from build123d import *

# Parameters (mm, degrees)
SKETCH1_W           = 18
SKETCH1_H           = 18
SKETCH1_R           = 5
BOSS_EXTRUDE1_DEPTH = 18
SKETCH2_R           = 5
CUT_EXTRUDE1_DEPTH  = 3


with BuildPart() as part:
    # Sketch1 → Boss-Extrude1 (new body)
    with BuildSketch(Plane.XY):
        Rectangle(SKETCH1_W, SKETCH1_H)
        Circle(SKETCH1_R, mode=Mode.SUBTRACT)
    extrude(amount=BOSS_EXTRUDE1_DEPTH)

    # Sketch2 → Cut-Extrude1 (cut)
    with BuildSketch(Plane(origin=(9, 0, 0), x_dir=(0, 0, -1), z_dir=(1, 0, 0))):
        with Locations(Location((-9, 0, 0), (0, 0, 90))):
            Circle(SKETCH2_R)
    cut_extrude1 = extrude(amount=-CUT_EXTRUDE1_DEPTH, mode=Mode.SUBTRACT)

    # Mirror1: Cut-Extrude1 across plane
    add(cut_extrude1.mirror(Plane(origin=(0, 0, 0), x_dir=(0, 0, 1), z_dir=(1, 0, 0))), mode=Mode.SUBTRACT)


solid = part.part
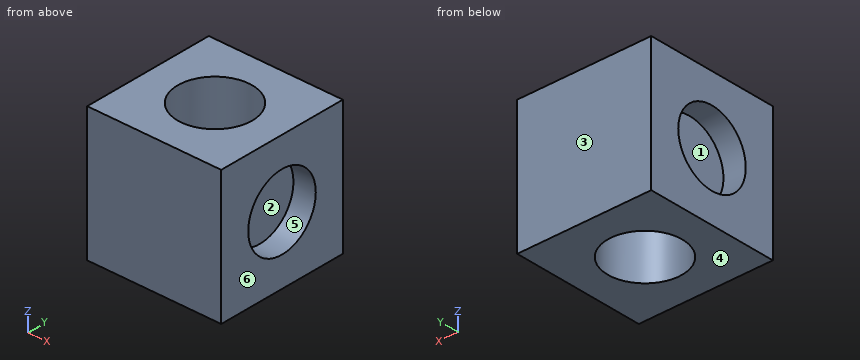
Source: CAD feature listing. Evaluate the final solid. Frame: model axes, mm. Face numbers are marked on the shaded views. A direction names the side the tool comes from. Round coordinates to 2 decimals unless told otherwise and drop trailing zeros. Loops run counter-clockwise (first coordinate to the right, second up) from the corner with the lowest first, then second, coordinate; pieces in that order, holes last.
Q1. Mould query, pull axis Z, two halves, no side actions, for the marked faces 4, 5 and 6. Classes: pulls with the +Z half, pulls with the -Z half, needs draft (parallel to the pull), parting line crosses it, or undercut.
Q2. Section B-B, the plane y = 0. Return loops of the section in (x, z), plus the area to 3 significant figures.
Q3. Section D-D, the plane x = 4. Return loops of the section in (y, z), plus the area to 3 significant figures.
Q4. Access query for the marked faces 1, 2 and 3. Directions: +Z, -Z, +X, -X, +Y, -Y. A direction counts if a zero-diameter tool reaches every point of the face in a straight line with its end or side. Return the directions, or none.
Q5. Section C-C, the plane z = 5. Return loops of the section in (x, y).
Q6. Section A-A, the plane x = 0. Return loops of the section in (y, z).
Q7. Ray query, line 1 (Z direction, x = -7.2, y = 0); line 2 (Y direction, x = 0, z = 4.5); line 3 (Y direction, x = -2.5, z = 2). Return the intervals inside material, ascending.
Q8. First-contact query: P1, Ø1.5, axis at y = -0.5, z = 13, coming from the -X side; P2, Ø3, axis at y = 0.5, z = 9, coming from the +X side. Flat tips, straight axial feed; report the tip coordinate or a pass-through.
Solutions:
1. face 4: pulls with the -Z half
1. face 5: undercut
1. face 6: needs draft
2. outline: (-9, 0) - (-5, 0) - (-5, 18) - (-9, 18) - (-9, 14) - (-6, 14) - (-6, 4) - (-9, 4) - close; (5, 0) - (9, 0) - (9, 4) - (6, 4) - (6, 14) - (9, 14) - (9, 18) - (5, 18) - close
2. area: 84.0 mm2
3. outline: (-9, 0) - (-3, 0) - (-3, 18) - (-9, 18) - close; (3, 0) - (9, 0) - (9, 18) - (3, 18) - close
3. area: 216 mm2
4. face 1: -X
4. face 2: +X
4. face 3: +Z, -Z, +X, -X, +Y
5. outline: (-9, -9) - (9, -9) - (9, -3) - (6, -3) - (6, 3) - (9, 3) - (9, 9) - (-9, 9) - (-9, 3) - (-6, 3) - (-6, -3) - (-9, -3) - close; hole circle Ø10 at (0, 0)
6. outline: (-9, 0) - (-5, 0) - (-5, 18) - (-9, 18) - close; (5, 0) - (9, 0) - (9, 18) - (5, 18) - close
7. line 1: z = 0 to 4, 14 to 18
7. line 2: y = -9 to -5, 5 to 9
7. line 3: y = -9 to -4.33, 4.33 to 9
8. P1: stops at x = -6
8. P2: stops at x = 6
